Print and shaded views of the part. All mm, measured from the part's lowest x, y and z. A direction names the side the tool comes from. Round coordinates to 2 decimals unless told otherwise and drop trailing zeros. Order: outer loops, then holes, each group sorted by start corner. A loop starts at its lowest first (then second) coordinate and runs counter-clockwise, first axis right, second up. Notation, with made-up numbers: (-5.5, 54.5) -> (48.5, 54.5) arc R32 ccw to (48.5, 93.5) -> close; hole circle Ø10 at (-37.75, 82). An arc over 180 degrees is marked (long way). Answer as CSV lines item,"result".
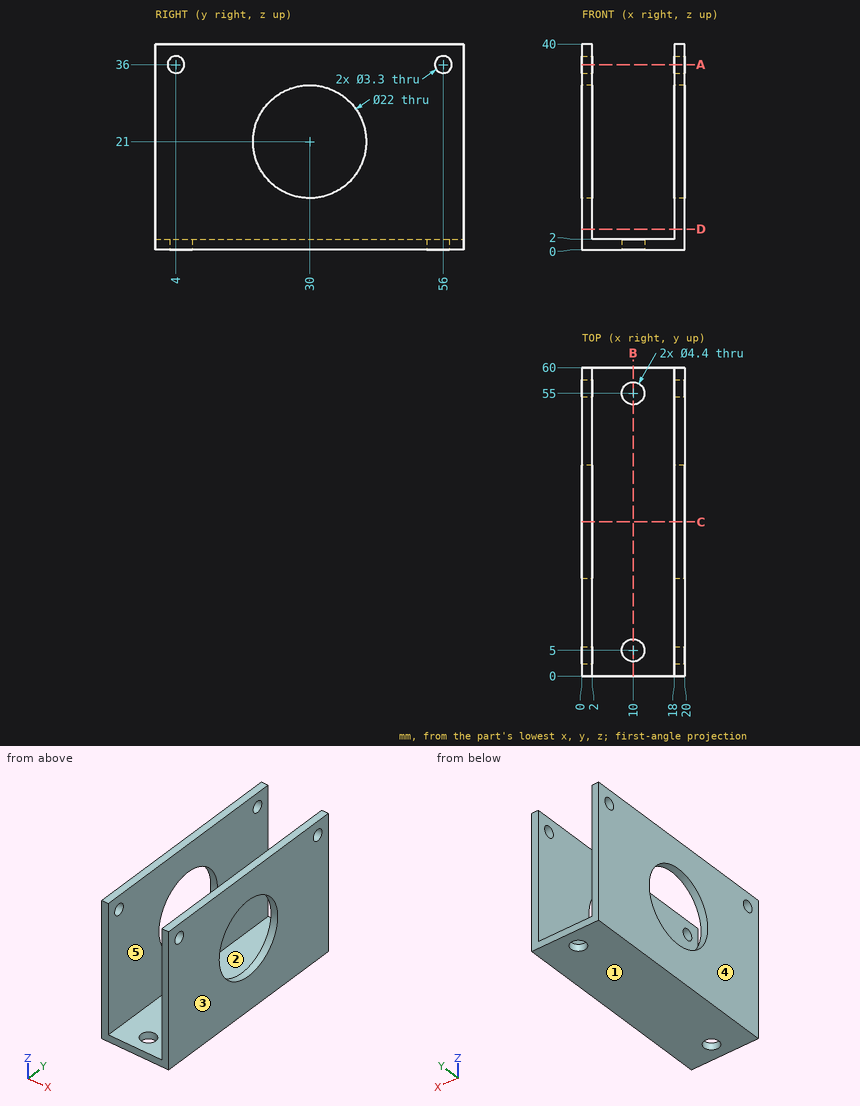
Q1. Mould opens along X. For the marked faces 3, 4 and 5 say: +X half, -X half, draft (parallel to the pull), parting line (faces both ways), or undercut.
Checks:
face 3,"+X half"
face 4,"-X half"
face 5,"undercut"
Q2. Flat gauge pins, fed straight in: pin 1 (4 mm diameter, centred on y = 4, z = 36, fed in from -X); pin 2 (6 mm diameter, centred on x = 14.5, y = 33.5, fed in from +Z). Where does each tip first touch, or does it go through?
Checks:
pin 1,"x = 0"
pin 2,"z = 2"
Q3. Wall check: L1, parallel to Y at x = 10, z = 0.55; L2, parallel to X at y = 20, z = 35.5; L3, parallel to Z at x = 0.55, y = 56. Give the ranges that are in metal, low to high. Write a range as [from, to].
Checks:
L1,"[0, 2.8], [7.2, 52.8], [57.2, 60]"
L2,"[0, 2], [18, 20]"
L3,"[0, 34.35], [37.65, 40]"
Q4. Tool access for the marked faces 1 and 2: list every direction of +Z, -Z, +X, -X, +Y, -Y with a clear straight run to the whole face (end or side of a thin tool).
Checks:
face 1,"-Z, +X, -X, +Y, -Y"
face 2,"+Z, +Y, -Y"
Q5. Saw through at B-B (x = 10). Write the cut outline in (y, z), plus the area to 3 significant figures.
Checks:
outline,"(0, 0) -> (2.8, 0) -> (2.8, 2) -> (0, 2) -> close; (7.2, 0) -> (52.8, 0) -> (52.8, 2) -> (7.2, 2) -> close; (57.2, 0) -> (60, 0) -> (60, 2) -> (57.2, 2) -> close"
area,"102 mm²"
Q6. Saw through at D-D (z = 4). Write the cut outline in (x, y).
Checks:
outline,"(0, 0) -> (2, 0) -> (2, 60) -> (0, 60) -> close; (18, 0) -> (20, 0) -> (20, 60) -> (18, 60) -> close"
Q7. Saw through at C-C (y = 30). Write the cut outline in (x, z).
Checks:
outline,"(0, 0) -> (20, 0) -> (20, 10) -> (18, 10) -> (18, 2) -> (2, 2) -> (2, 10) -> (0, 10) -> close; (0, 32) -> (2, 32) -> (2, 40) -> (0, 40) -> close; (18, 32) -> (20, 32) -> (20, 40) -> (18, 40) -> close"
Q8. Saw through at A-A (z = 36). Write the cut outline in (x, y), plus the area to 3 significant figures.
Checks:
outline,"(0, 0) -> (2, 0) -> (2, 2.35) -> (0, 2.35) -> close; (0, 5.65) -> (2, 5.65) -> (2, 54.35) -> (0, 54.35) -> close; (0, 57.65) -> (2, 57.65) -> (2, 60) -> (0, 60) -> close; (18, 0) -> (20, 0) -> (20, 2.35) -> (18, 2.35) -> close; (18, 5.65) -> (20, 5.65) -> (20, 54.35) -> (18, 54.35) -> close; (18, 57.65) -> (20, 57.65) -> (20, 60) -> (18, 60) -> close"
area,"214 mm²"
